Check sheet for the drawn part. Datum: minimum x, y, z corner. Units: mm. Round coordinates to 2 decimals unless told otherwise and drop trailing zeros. Write each loop counter-clockwise with the first axis right and the second up, starting at its lowest first coordinate (ties: lowest second). Pieces come first, ordered by that corner, then holes. Notation, with made-up numbers: (-39, -37.75) - (-11, -37.75) arc R18 ccw to (-11, -27.75) - close; hole circle Ø1 at (2.5, 27). An arc over 180 degrees is marked (long way). Write each question's results on one line, items separated by ' | '.
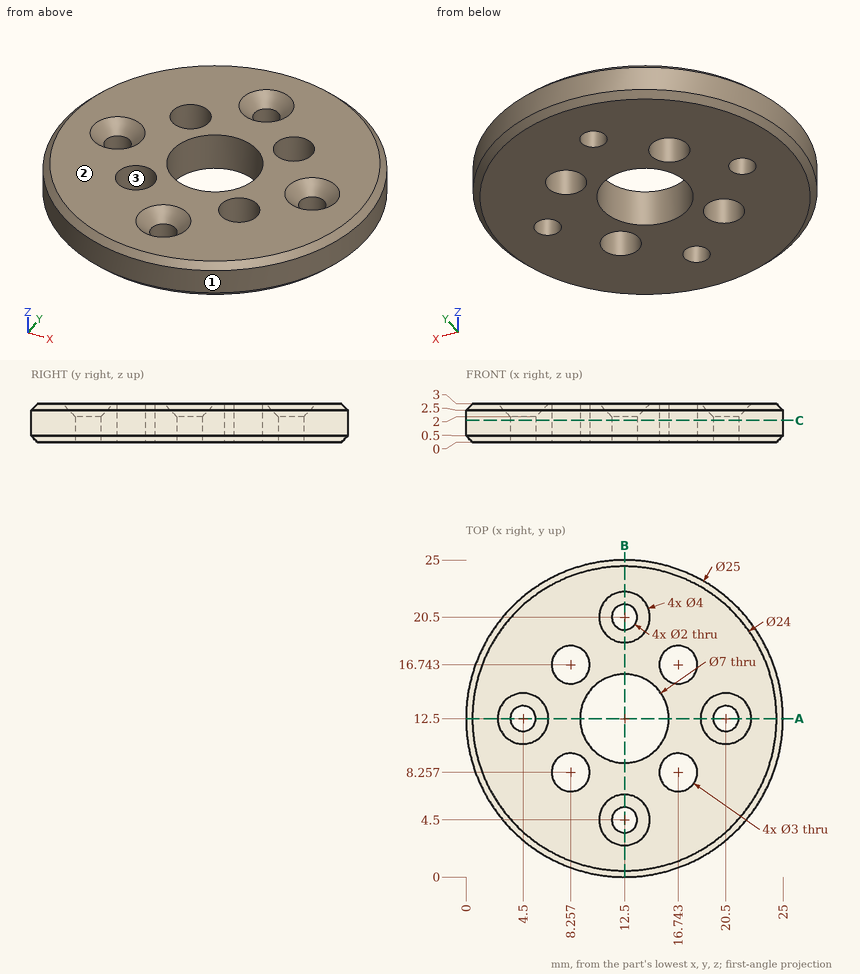
(1) Section check C-C (z = 1.7). State how many separate pieces and enclosed holes the cut face has.
Answer:
separate pieces: 1 | enclosed holes: 9
(2) Mould release check, pull along X, two halves, no side actions. Record for the marked faces 1, 2 and 3: released by +X, released by -X, zero draft, split by the parting line, or undercut.
Answer:
face 1: split by the parting line | face 2: zero draft | face 3: undercut
(3) Thickness scan on L1, parallel to Y at x = 7, z = 2.05 (1 decimal); L2, parallel to Y at x = 15.5, z = 1.25 (1 decimal); L3, parallel to X at y = 8.5, z = 1.4. Record the ranges inside material, lowest first.
Answer:
L1: 1.3 to 7.4, 9.1 to 15.9, 17.6 to 23.7 | L2: 0.4 to 7.4, 9.1 to 10.7, 14.3 to 15.9, 17.6 to 24.6 | L3: 0.66 to 6.78, 9.74 to 15.26, 18.22 to 24.34
(4) Section check A-A (y = 12.5). Record the cut outline in (x, z), plus the area to 3 significant figures.
Answer:
outline: (0, 0.5) - (0.5, 0) - (3.5, 0) - (3.5, 2) - (2.5, 3) - (0.5, 3) - (0, 2.5) - close; (5.5, 0) - (9, 0) - (9, 3) - (6.5, 3) - (5.5, 2) - close; (16, 0) - (19.5, 0) - (19.5, 2) - (18.5, 3) - (16, 3) - close; (21.5, 0) - (24.5, 0) - (25, 0.5) - (25, 2.5) - (24.5, 3) - (22.5, 3) - (21.5, 2) - close | area: 39.5 mm2
(5) Go/stop test with flat-tipped pins: pin 1 Ø1 at (x, z) = (17, 1) entering from +Y; pin 2 Ø2.5 at (x, y) = (16.74, 8.26) entering from -Z; pin 3 Ø1.5 at (x, z) = (21, 0.5) entering from -Y; pin 4 Ø1 at (y, z) = (19, 1.5) entering from +X (1 decimal). Record where each tip stops, or that it passes through.
Answer:
pin 1: y = 24.34 | pin 2: through | pin 3: y = 2.69 | pin 4: x = 23.5
